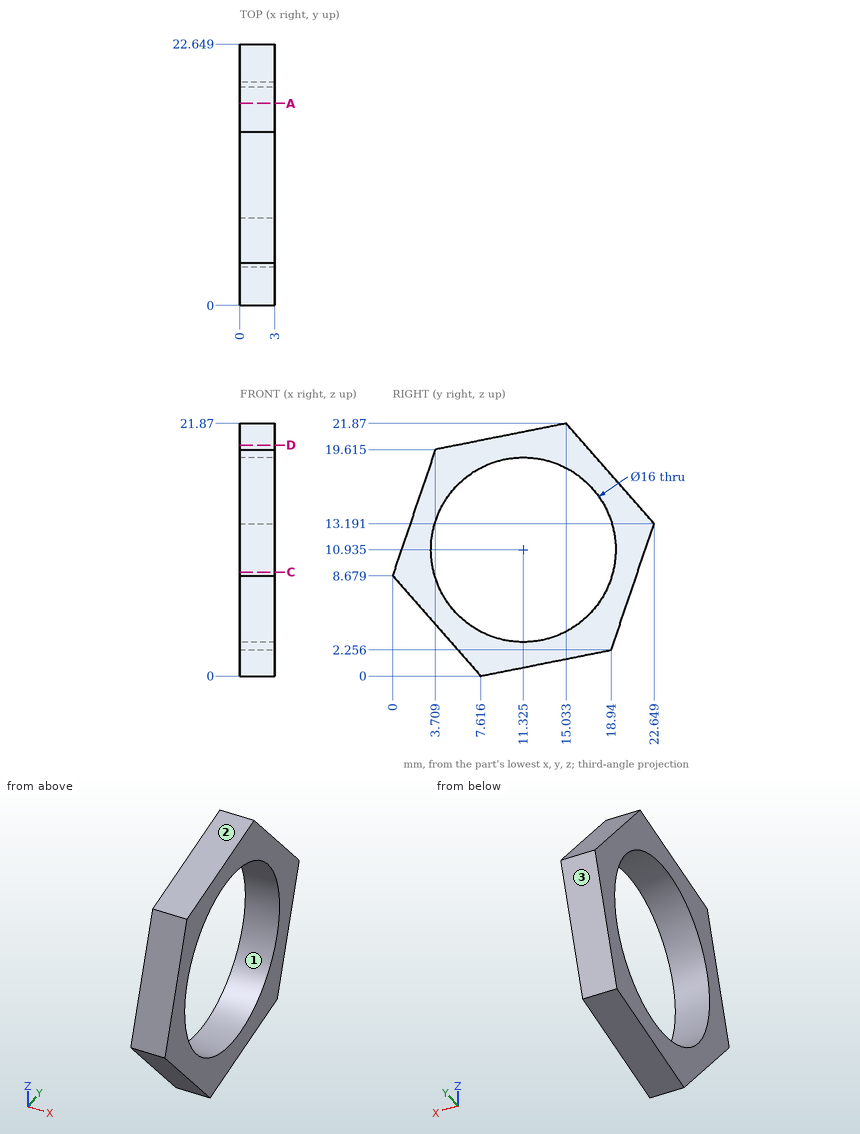
Geometry check sheet. Reference: drawing and pictorial views, mm from the part's lowest x, y, z. Round coordinates to 2 decimals unless told otherwise and drop trailing zeros. Order: outer loops, then holes, each group sorted by start corner. A loop starts at its lowest first (then second) coordinate and runs counter-clockwise, first axis right, second up. Notation, with made-up numbers: (-13, 8.25) -> (16, 8.25) arc R18 ccw to (16, 12.25) -> close; hole circle Ø6 at (40.5, -30). An arc over 180 degrees is marked (long way). One line per item, written item: value. Start each with the question number.
Q1. Thickness scan on line 1 (Z direction, x = 0.8, y = 12) (1 decimal); line 2 (Z direction, x = 2.15, y = 7.5) (1 decimal); line 3 (Y direction, x = 1.1, z = 8) (1 decimal). Record the ranges inside material, lowest first.
Q2. Gauge pin test, flat end, axial feed: pin 1 Ø1 at (x, z) = (1, 10) entering from +Y. Record the tip position at first contact, or that the pin passes through.
Q3. Cross-section at D-D (z = 20). Record the boundary of the cut face in (x, y) (1 decimal).
Q4. Mould release check, pull along Z, two halves, no side actions. Record for the marked faces 1, 2 and 3: pulls with the +Z half, pulls with the -Z half, needs draft (parallel to the pull), parting line crosses it, or undercut.
Q5. Cross-section at A-A (y = 17.5). Record the boundary of the cut face in (x, z).
Q6. Cross-section at C-C (z = 9). Record the boundary of the cut face in (x, y).
Completed:
1. line 1: z = 0.9 to 3, 18.9 to 21.3
1. line 2: z = 0.1 to 3.9, 18 to 20.4
1. line 3: y = 0.6 to 3.9, 18.8 to 20.9
2. pin 1: stops at y = 21.74
3. outline: (0, 5.6) -> (3, 5.6) -> (3, 16.7) -> (0, 16.7) -> close
4. face 1: undercut
4. face 2: pulls with the +Z half
4. face 3: pulls with the -Z half
5. outline: (0, 1.97) -> (3, 1.97) -> (3, 5.85) -> (0, 5.85) -> close; (0, 16.02) -> (3, 16.02) -> (3, 19.06) -> (0, 19.06) -> close
6. outline: (0, 0.11) -> (3, 0.11) -> (3, 3.56) -> (0, 3.56) -> close; (0, 19.09) -> (3, 19.09) -> (3, 21.23) -> (0, 21.23) -> close
